```python
from build123d import *

# Parameters (mm, degrees)
SKETCH1_R          = 1.01901554
EXTRUDE1_DEPTH     = 1
SKETCH2_R          = 1.5
CUT_EXTRUDE2_DEPTH = 29.071089649
FILLET1_R          = 1


with BuildPart() as part:
    # Sketch1 → Extrude1 (new body)
    with BuildSketch(Plane.XY):
        with BuildLine():
            Line((0, 2.038031079), (-25.941113, 2.038031079))
            ThreePointArc((-25.941113, 2.038031079), (-27.979144079, 0), (-25.941113, -2.038031079))
            Line((-25.941113, -2.038031079), (0, -2.038031079))
            ThreePointArc((0, -2.038031079), (2.038031079, 0), (0, 2.038031079))
        make_face()
        with Locations((-25.941113, 0)):
            Circle(SKETCH1_R, mode=Mode.SUBTRACT)
        Circle(SKETCH1_R, mode=Mode.SUBTRACT)
    extrude(amount=EXTRUDE1_DEPTH)

    # Sketch2 → Cut-Extrude2 (cut, through all)
    with BuildSketch(Plane.XY):
        with Locations((-2.302162805, 2.3)):
            Circle(SKETCH2_R)
    extrude(amount=CUT_EXTRUDE2_DEPTH, mode=Mode.SUBTRACT)

    # Fillet1
    fillet1_edges = [part.edges().sort_by_distance(p)[0] for p in [
        (-0.825215858, 2.038031079, 0.5),
        (-3.779109752, 2.038031079, 0.5),
    ]]
    fillet(fillet1_edges, radius=FILLET1_R)


solid = part.part
```
CAD build for the part. Positions are in the model's coordinates, mm. A direction names the side the tool comes from. Round coordinates to 2 decimals unless told otherwise and drop trailing zeros. Order: outer loops, then holes, each group sorted by start corner. A loop starts at its lowest first (then second) coordinate and runs counter-clockwise, first axis right, second up.
Item 1: Probe line 1 along X through (y, z) = (0.1, 0.95); line 2 along X through (y, z) = (-0.45, 0.75); line 3 along X through (y, z) = (-1.4, 0.4). List the from-to ranges inside material, lowest first.
Item 2: Saw through at A-A on z = 0.65. Write the cut outline in (x, y), then the cut area to 3 significant figures.
Item 3: Saw through at D-D on y = -1.4. Write the cut outline in (x, z).
Item 4: Saw through at B-B on y = 0. Write the cut outline in (x, z).
Item 5: Tool access for faces 5 (the face through (-3.956, 1.902, 0.493)), 6 (the face through (-13.2, -2.038, 0.5)): list every direction of +Z, -Z, +X, -X, +Y, -Y with a clear straight run to the whole face (end or side of a thin tool).
Item 6: Mould opens along X. For faces 1 (the face through (-0.13, 1.01, 0.49)), 2 (the face through (-2.3, 0.8, 0.5)), 3 (the face through (-13, 0, 1)), 4 (the face through (2.038, -0.045, 0.493)) say: pulls with the +X half, pulls with the -X half, needs draft (parallel to the pull), parting line crosses it, or undercut.
Item 7: Saw through at C-C on y = 1.3. Write the cut outline in (x, z).
Reported:
1. line 1: x = -27.98 to -26.96, -24.93 to -1.01, 1.01 to 2.04
1. line 2: x = -27.93 to -26.86, -25.03 to -0.91, 0.91 to 1.99
1. line 3: x = -27.42 to 1.48
2. outline: (-25.94, -2.04) - (0, -2.04) arc R2.04 ccw to (0, 2.04) - (-0.14, 2.04) arc R1 ccw to (-1.01, 1.54) arc R1.5 cw to (-3.6, 1.54) arc R1 ccw to (-4.46, 2.04) - (-25.94, 2.04) arc R2.04 ccw to start; hole circle Ø2.04 at (-25.94, 0); hole circle Ø2.04 at (0, 0)
2. area: 109 mm2
3. outline: (-27.42, 0) - (1.48, 0) - (1.48, 1) - (-27.42, 1) - close
4. outline: (-27.98, 0) - (-26.96, 0) - (-26.96, 1) - (-27.98, 1) - close; (-24.92, 0) - (-1.02, 0) - (-1.02, 1) - (-24.92, 1) - close; (1.02, 0) - (2.04, 0) - (2.04, 1) - (1.02, 1) - close
5. face 5: +Z, -Z, +Y
5. face 6: +Z, -Z, +X, -X, -Y
6. face 1: undercut
6. face 2: undercut
6. face 3: needs draft
6. face 4: pulls with the +X half
7. outline: (-27.51, 0) - (-3.42, 0) - (-3.42, 1) - (-27.51, 1) - close; (-1.18, 0) - (1.57, 0) - (1.57, 1) - (-1.18, 1) - close
